```python
from build123d import *

# Parameters (mm, degrees)
ESQUISSE1_R             = 37
BOSS_EXTRU_1_DEPTH      = 6
ESQUISSE2_R             = 35
ENL_V_MAT_EXTRU_1_DEPTH = 4
CONG_1_R                = 2


with BuildPart() as part:
    # Esquisse1 → Boss.-Extru.1 (new body)
    with BuildSketch(Plane.XY):
        Circle(ESQUISSE1_R)
    extrude(amount=BOSS_EXTRU_1_DEPTH)

    # Esquisse2 → Enlèv. mat.-Extru.1 (cut)
    with BuildSketch(Plane.XY.offset(6)):
        Circle(ESQUISSE2_R)
    extrude(amount=-ENL_V_MAT_EXTRU_1_DEPTH, mode=Mode.SUBTRACT)

    # Congé1
    cong_1_edges = [part.edges().sort_by_distance(p)[0] for p in [
        (-37, 0, 0),
    ]]
    fillet(cong_1_edges, radius=CONG_1_R)


solid = part.part
```
Geometry check sheet. Reference: the model listing, model coordinates, mm. Coordinates: 2 decimals unless noted, no trailing zeros. Write each loop counter-clockwise with the first axis right and the second up, starting at its lowest first coordinate (ties: lowest second). Pieces come first, ordered by that corner, then holes. Notation, with made-up numbers: (55.5, 85.5) -> (73.5, 85.5) arc R23 ccw to (73.5, 113.5) -> close; hole circle Ø11 at (26.25, 70.25). An arc over 180 degrees is marked (long way). Use CSV: the item, a comma, the result in double quotes. Start each with the question number.
Item 1: Cross-section at A-A, the plane x = 0. Record the cut outline in (y, z).
Item 2: Depth check by flat-ended pin: pin 1 Ø3 at (x, z) = (7, 5) entering from +Y; pin 2 Ø6 at (x, y) = (6, -26.5) entering from +Z; pin 3 Ø2 at (y, z) = (10.5, 3.5) entering from +X. Enter the tip coordinate at first touch or a pass-through.
Item 3: Mould release check, pull along Y, two halves, no side actions. Record for faces 1 (the flat face through (0, 0, 2)), 2 (the cylindrical face through (-28, -21, 4)), 3 (the cylindrical face through (-8.02, -36.12, 3.97)), 4 (the flat face through (0, 0, 0)): released by +Y, released by -Y, zero draft, split by the parting line, or undercut.
Item 4: Thickness scan on line 1 (Z direction, x = 19.5, y = 13); line 2 (Y direction, x = -3.5, z = 3.1); line 3 (Y direction, x = -12.5, z = 2.6). Record the ranges inside material, lowest first.
Answers:
1,outline,"(-37, 2) arc R2 ccw to (-35, 0) -> (35, 0) arc R2 ccw to (37, 2) -> (37, 6) -> (35, 6) -> (35, 2) -> (-35, 2) -> (-35, 6) -> (-37, 6) -> close"
2,pin 1,"y = 36.59"
2,pin 2,"z = 2"
2,pin 3,"x = 35.76"
3,face 1,"undercut"
3,face 2,"undercut"
3,face 3,"split by the parting line"
3,face 4,"zero draft"
4,line 1,"0 to 2"
4,line 2,"-36.83 to -34.82, 34.82 to 36.83"
4,line 3,"-34.82 to -32.69, 32.69 to 34.82"
